Design review of the part built by this model. Coordinates are the model's own, in mm. Face numbers are marked on the shaded views. A direction names the side the tool comes from. Give positions to 0.01 mm unless a question says otherwise; leave off trailing zeros. Loops run counter-clockwise (first coordinate to the right, second up) from the corner with the lowest first, then second, coordinate; pieces in that order, holes last. Notation, with made-up numbers: (8, -3.5) -> (15, -3.5) arc R28 ccw to (15, 20.5) -> close; hole circle Ø9 at (79.5, 58.25). An arc over 180 degrees is marked (long way). Answer in a Markdown table with one row per item. Add a question column.
(1) For the marked faces 5 and 6, list the 3-axis set-ups (+Z, -Z, +X, -X, +Y, -Y) from which the entire face can be reached by the end or side of a thin tool; tool diameter is ignored.
(2) Consider section A-A on z = 17.2. Write out the cut boundary in (x, y).
(3) Consider section D-D on y = 16.5. Count the separate pieces of the cut face and the enclosed holes in it, then the cut area to 3 significant figures.
(4) Consider section C-C on y = -4. Write out the cut boundary in (x, z).
(5) Draft analysis for pull direction X (two halves, no side actions). For the marked faces 1, 2, 3 and 4, state which applies: +X half, -X half, draft (parallel to the pull), parting line (faces both ways), or undercut.
(6) Consider section B-B on x = 4.5. Write out the cut boundary in (y, z).
(7) For pin 1 (3.5 mm diameter, centred on x = 16.5, z = 62, fed in from +Y); pin 2 (3 mm diameter, centred on y = 16.5, z = 24.5, fed in from -X) (3 decimals); pin 3 (3 mm diameter, centred on x = -1, z = 10.5, fed in from -Y), all flat-tipped, find the tip position at first contact; note any pin that passes through.
(8) For line 1 (Y direction, x = -15, z = 61); line 2 (X direction, y = -17, z = 62); line 3 (Y direction, x = -16.7, z = 24.5), list the stretches that pass through material, from the lowest coordinate up.
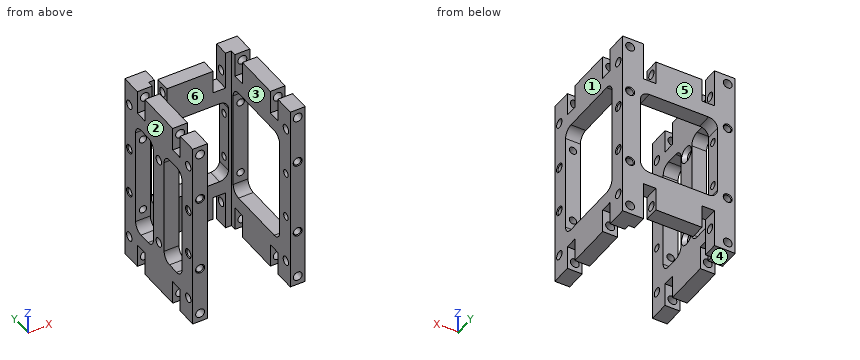
from build123d import *

# Parameters (mm, degrees)
EXTRUDE_1_DEPTH                = 65
SKETCH_2_R                     = 1.5
SKETCH_2_R_2                   = 1.25
SKETCH_2_W                     = 8
SKETCH_2_H                     = 4.2
SKETCH_2_W_2                   = 39
SKETCH_2_H_2                   = 26
CUT_EXTRUDE_1_DEPTH            = 78.653074633
SKETCH_3_R                     = 1.5
SKETCH_3_R_2                   = 1.25
SKETCH_3_W                     = 26
SKETCH_3_H                     = 29
CUT_EXTRUDE_2_DEPTH            = 60
SKETCH_5_W                     = 39
SKETCH_5_H                     = 6
SKETCH_5_R                     = 1.5
EXTRUDE_2_DEPTH                = 5
FILLET_1_R                     = 3
HOLE_WIZARD_M3_1_9_D           = 3
HOLE_WIZARD_M3_1_9_CSINK_D     = 5.5
HOLE_WIZARD_M3_1_9_CSINK_ANGLE = 90


# Read off the part's stored shape, not the designer's step: M3 螺纹孔1
with BuildPart() as part:
    # 草图1 → 凸台-拉伸1 (new body)
    with BuildSketch(Plane.XY):
        Polygon((-14, -19), (-14, 14), (14, 14), (14, -19), (19, -19), (19, 19), (-19, 19), (-19, -19), align=None)
    extrude(amount=EXTRUDE_1_DEPTH)

    # 草图2 → 切除-拉伸1 (cut, through all)
    with BuildSketch(Plane.ZY.offset(19)):
        with Locations(Location((57, -16.5, 0), (0, 0, 270))):
            Circle(SKETCH_2_R)
        with Locations(Location((57, 16.5, 0), (0, 0, 270))):
            Circle(SKETCH_2_R)
        with Locations(Location((8, -16.5, 0), (0, 0, 90))):
            Circle(SKETCH_2_R)
        with Locations(Location((8, 16.5, 0), (0, 0, 90))):
            Circle(SKETCH_2_R)
        with Locations(Location((40.5, -16.5, 0), (0, 0, 270))):
            Circle(SKETCH_2_R_2)
        with Locations(Location((24.5, -16.5, 0), (0, 0, 270))):
            Circle(SKETCH_2_R_2)
        with Locations(Location((24.5, 16.5, 0), (0, 0, 90))):
            Circle(SKETCH_2_R_2)
        with Locations(Location((40.5, 16.5, 0), (0, 0, 90))):
            Circle(SKETCH_2_R_2)
        with Locations((61, 9.9)):
            Rectangle(SKETCH_2_W, SKETCH_2_H)
        with Locations((61, -9.9)):
            Rectangle(SKETCH_2_W, SKETCH_2_H)
        with Locations((4, -9.9)):
            Rectangle(SKETCH_2_W, SKETCH_2_H)
        with Locations((4, 9.9)):
            Rectangle(SKETCH_2_W, SKETCH_2_H)
        with Locations((32.5, 0)):
            Rectangle(SKETCH_2_W_2, SKETCH_2_H_2)
    extrude(amount=-CUT_EXTRUDE_1_DEPTH, mode=Mode.SUBTRACT)

    # 草图3 → 切除-拉伸2 (cut)
    with BuildSketch(Plane(origin=(0, 19, 0), x_dir=(1, 0, 0), z_dir=(0, 1, 0))):
        with Locations(Location((16.5, -62, 0), (0, 0, 270))):
            Circle(SKETCH_3_R)
        with Locations(Location((-16.5, -62, 0), (0, 0, 270))):
            Circle(SKETCH_3_R)
        with Locations(Location((-16.5, -3, 0), (0, 0, 270))):
            Circle(SKETCH_3_R)
        with Locations(Location((16.5, -3, 0), (0, 0, 180))):
            Circle(SKETCH_3_R)
        with Locations(Location((16.5, -45.5, 0), (0, 0, 270))):
            Circle(SKETCH_3_R_2)
        with Locations(Location((16.5, -19.5, 0), (0, 0, 270))):
            Circle(SKETCH_3_R_2)
        with Locations(Location((-16.5, -19.5, 0), (0, 0, 270))):
            Circle(SKETCH_3_R_2)
        with Locations(Location((-16.5, -45.5, 0), (0, 0, 180))):
            Circle(SKETCH_3_R_2)
        Polygon((7.8, -65), (-7.8, -65), (-12, -65), (-12, -52), (-7.8, -52), (-7.8, -60), (7.8, -60), (7.8, -52), (12, -52), (12, -65), align=None)
        Polygon((-12, 0), (-12, -13), (-7.8, -13), (-7.8, -5), (7.8, -5), (7.8, -13), (12, -13), (12, 0), (7.8, 0), (-7.8, 0), align=None)
        with Locations((0, -32.5)):
            Rectangle(SKETCH_3_W, SKETCH_3_H)
    extrude(amount=-CUT_EXTRUDE_2_DEPTH, mode=Mode.SUBTRACT)

    # Hole Wizard M3 _1 outline → Hole Wizard M3 _1 (revolve, cut)
    with BuildSketch(Plane(origin=(0, 16.5, 24.5), x_dir=(0, 1, 0), z_dir=(0, 0, -1))):
        Polygon((1.25, 19), (1.25, 18.725), (1.525, 19), align=None)
        Polygon((1.525, -19), (1.25, -18.725), (1.25, -19), align=None)
    revolve(axis=Axis((0, 16.5, 24.5), (1, 0, 0)), mode=Mode.SUBTRACT)

    # Hole Wizard M3 _1 2 outline → Hole Wizard M3 _1 2 (revolve, cut)
    with BuildSketch(Plane(origin=(0, 16.5, 40.5), x_dir=(0, 1, 0), z_dir=(0, 0, -1))):
        Polygon((1.25, 19), (1.25, 18.725), (1.525, 19), align=None)
        Polygon((1.525, -19), (1.25, -18.725), (1.25, -19), align=None)
    revolve(axis=Axis((0, 16.5, 40.5), (1, 0, 0)), mode=Mode.SUBTRACT)

    # Hole Wizard M3 _1 3 outline → Hole Wizard M3 _1 3 (revolve, cut)
    with BuildSketch(Plane(origin=(0, -16.5, 40.5), x_dir=(0, 1, 0), z_dir=(0, 0, -1))):
        Polygon((1.25, 19), (1.25, 18.725), (1.525, 19), align=None)
        Polygon((1.525, -19), (1.25, -18.725), (1.25, -19), align=None)
    revolve(axis=Axis((0, -16.5, 40.5), (1, 0, 0)), mode=Mode.SUBTRACT)

    # Hole Wizard M3 _1 4 outline → Hole Wizard M3 _1 4 (revolve, cut)
    with BuildSketch(Plane(origin=(0, -16.5, 24.5), x_dir=(0, 1, 0), z_dir=(0, 0, -1))):
        Polygon((1.25, 19), (1.25, 18.725), (1.525, 19), align=None)
        Polygon((1.525, -19), (1.25, -18.725), (1.25, -19), align=None)
    revolve(axis=Axis((0, -16.5, 24.5), (1, 0, 0)), mode=Mode.SUBTRACT)

    # Hole Wizard M3 _1 5 outline → Hole Wizard M3 _1 5 (revolve, cut)
    with BuildSketch(Plane(origin=(16.5, 0, 45.5), x_dir=(1, 0, 0), z_dir=(0, 0, 1))):
        Polygon((1.525, -19), (1.25, -18.725), (1.25, -19), align=None)
        Polygon((1.25, 19), (1.25, 18.725), (1.525, 19), align=None)
    revolve(axis=Axis((16.5, 0, 45.5), (0, 1, 0)), mode=Mode.SUBTRACT)

    # Hole Wizard M3 _1 6 outline → Hole Wizard M3 _1 6 (revolve, cut)
    with BuildSketch(Plane(origin=(-16.5, 0, 19.5), x_dir=(1, 0, 0), z_dir=(0, 0, 1))):
        Polygon((1.525, -19), (1.25, -18.725), (1.25, -19), align=None)
        Polygon((1.25, 19), (1.25, 18.725), (1.525, 19), align=None)
    revolve(axis=Axis((-16.5, 0, 19.5), (0, 1, 0)), mode=Mode.SUBTRACT)

    # Hole Wizard M3 _1 7 outline → Hole Wizard M3 _1 7 (revolve, cut)
    with BuildSketch(Plane(origin=(-16.5, 0, 45.5), x_dir=(1, 0, 0), z_dir=(0, 0, 1))):
        Polygon((1.525, -19), (1.25, -18.725), (1.25, -19), align=None)
        Polygon((1.25, 19), (1.25, 18.725), (1.525, 19), align=None)
    revolve(axis=Axis((-16.5, 0, 45.5), (0, 1, 0)), mode=Mode.SUBTRACT)

    # Hole Wizard M3 _1 8 outline → Hole Wizard M3 _1 8 (revolve, cut)
    with BuildSketch(Plane(origin=(16.5, 0, 19.5), x_dir=(1, 0, 0), z_dir=(0, 0, 1))):
        Polygon((1.525, -19), (1.25, -18.725), (1.25, -19), align=None)
        Polygon((1.25, 19), (1.25, 18.725), (1.525, 19), align=None)
    revolve(axis=Axis((16.5, 0, 19.5), (0, 1, 0)), mode=Mode.SUBTRACT)

    # 草图5 → 凸台-拉伸2 (add)
    with BuildSketch(Plane.ZY.offset(19)):
        with Locations((32.5, 0)):
            Rectangle(SKETCH_5_W, SKETCH_5_H)
        with Locations((17.2, 0)):
            Circle(SKETCH_5_R, mode=Mode.SUBTRACT)
        with Locations((47.8, 0)):
            Circle(SKETCH_5_R, mode=Mode.SUBTRACT)
    extrude(amount=-EXTRUDE_2_DEPTH)

    # 圆角1
    fillet_1_edges = [part.edges().sort_by_distance(p)[0] for p in [
        (13, 16.5, 47),
        (-13, 16.5, 18),
        (13, 16.5, 18),
        (-13, 16.5, 47),
        (-16.5, -3, 52),
        (-16.5, 3, 52),
        (-16.5, 3, 13),
        (-16.5, -3, 13),
        (-16.5, 13, 52),
        (16.5, 13, 52),
        (-16.5, -13, 52),
        (16.5, -13, 52),
        (-16.5, -13, 13),
        (16.5, -13, 13),
        (-16.5, 13, 13),
        (16.5, 13, 13),
    ]]
    fillet(fillet_1_edges, radius=FILLET_1_R)

    # Hole Wizard M3 _1 9 (through all)
    with Locations(Plane(origin=(-14, 0, 47.8), x_dir=(0, 1, 0), z_dir=(1, 0, 0))):
        with Locations((0, 0), (0, -30.6)):
            CounterSinkHole(HOLE_WIZARD_M3_1_9_D / 2, HOLE_WIZARD_M3_1_9_CSINK_D / 2, counter_sink_angle=HOLE_WIZARD_M3_1_9_CSINK_ANGLE)


solid = part.part
Values follow:
| question | item | result |
|---|---|---|
| 1 | face 5 | +Z, -Z, +X, -X, +Y |
| 1 | face 6 | +Z, -Z, -Y |
| 2 | outline | (-19, -19) -> (-14, -19) -> (-14, -13) -> (-19, -13) -> close; (-19, -3) -> (-14, -3) -> (-14, -2.75) -> (-15.25, -1.5) -> (-19, -1.5) -> close; (-19, 1.5) -> (-15.25, 1.5) -> (-14, 2.75) -> (-14, 3) -> (-19, 3) -> close; (-19, 13) -> (-14, 13) -> (-14, 14) -> (14, 14) -> (14, 13) -> (19, 13) -> (19, 19) -> (-19, 19) -> close; (14, -19) -> (19, -19) -> (19, -13) -> (14, -13) -> close |
| 3 | separate pieces | 10 |
| 3 | enclosed holes | 8 |
| 3 | area | 1,060 mm2 |
| 4 | outline | (-19, 0) -> (-14, 0) -> (-14, 13.76) -> (-19, 13.76) -> close; (-19, 51.24) -> (-14, 51.24) -> (-14, 65) -> (-19, 65) -> close; (14, 0) -> (19, 0) -> (19, 13) -> (14, 13) -> close; (14, 52) -> (19, 52) -> (19, 65) -> (14, 65) -> close; hole circle Ø3 at (-16.5, 3); hole circle Ø3 at (-16.5, 62); hole circle Ø3 at (16.5, 3); hole circle Ø3 at (16.5, 62) |
| 5 | face 1 | +X half |
| 5 | face 2 | -X half |
| 5 | face 3 | undercut |
| 5 | face 4 | draft |
| 6 | outline | (14, 5) -> (19, 5) -> (19, 18) -> (14, 18) -> close; (14, 47) -> (19, 47) -> (19, 60) -> (14, 60) -> close; hole circle Ø3 at (16.5, 8); hole circle Ø3 at (16.5, 57) |
| 7 | pin 1 | y = 19 |
| 7 | pin 2 | x = -18.975 |
| 7 | pin 3 | y = 14 |
| 8 | line 1 | -19 to -12, -7.8 to 7.8, 12 to 19 |
| 8 | line 2 | -19 to -18, -15 to -14, 14 to 15, 18 to 19 |
| 8 | line 3 | -19 to -17.75, -15.25 to -13, -3 to 3, 13 to 15.25, 17.75 to 19 |
